Part model, mm, in its own coordinate system. A direction names the side the tool comes from. Give positions to 0.01 mm unless a question says otherwise; leave off trailing zeros. Loops run counter-clockwise (first coordinate to the right, second up) from the corner with the lowest first, then second, coordinate; pieces in that order, holes last. Notation, with made-up numbers: (43.25, 84.5) -> (85.25, 84.5) arc R22 ccw to (85.25, 95.5) -> close; hole circle Ø4 at (-36.5, 14.5). An arc over 180 degrees is marked (long way). One line per question, with ' | ' between items.
```python
from build123d import *

# Parameters (mm, degrees)
F0_W     = 101.6
F0_H     = 50.8
F1_DEPTH = 457.2
F2_W     = 101.6
F2_H     = 50.8
F3_DEPTH = 914.4


with BuildPart() as f1:
    # F0 (on Front) → F1 (new body, symmetric)
    with BuildSketch(Plane.XZ):
        Rectangle(F0_W, F0_H)
    extrude(amount=F1_DEPTH, both=True)

    # F2 (on face) → F3 (join)
    with BuildSketch(Plane.YZ.offset(50.8)):
        with Locations((-406.4, 0)):
            Rectangle(F2_W, F2_H)
    extrude(amount=F3_DEPTH)


solid = f1.part
```
1) Pin check, flat tips, straight feed: P1, Ø10, axis at x = 349.5, z = 5.5, coming from the +Y side; P2, Ø15, axis at y = -149, z = 1, coming from the +X side. Stop position of each tip, or through.
Found:
P1: y = -355.6 | P2: x = 50.8
2) Saw through at C-C (y = 126.5). Give the cut face in (x, z), and give its area (3 significant figures).
Found:
outline: (-50.8, -25.4) -> (50.8, -25.4) -> (50.8, 25.4) -> (-50.8, 25.4) -> close | area: 5,160 mm2
3) Saw through at A-A (z = -7). Give the cut face in (x, y).
Found:
outline: (-50.8, -457.2) -> (965.2, -457.2) -> (965.2, -355.6) -> (50.8, -355.6) -> (50.8, 457.2) -> (-50.8, 457.2) -> close
4) Saw through at B-B (x = 248). Give the cut face in (y, z).
Found:
outline: (-457.2, -25.4) -> (-355.6, -25.4) -> (-355.6, 25.4) -> (-457.2, 25.4) -> close
5) Drill centre lines: line 1 (X direction, y = -183.5, z = 23.5); line 2 (Y direction, x = 390, z = -14.5). Where is each one in solid material? Low to high.
Found:
line 1: -50.8 to 50.8 | line 2: -457.2 to -355.6
6) Tool access for faces 1 (the flat face through (450, -457.2, 0)), 2 (the flat face through (502, -355.6, 0)): list every direction of +Z, -Z, +X, -X, +Y, -Y with a clear straight run to the whole face (end or side of a thin tool).
Found:
face 1: +Z, -Z, +X, -X, -Y | face 2: +Z, -Z, +X, +Y
